Check sheet for the drawn part. Datum: minimum x, y, z corner. Units: mm. A direction names the side the tool comes from. Round coordinates to 2 decimals unless told otherwise and drop trailing zeros. Order: outer loops, then holes, each group sorted by start corner. A loop starts at its lowest first (then second) coordinate and runs counter-clockwise, first axis right, second up. Notation, with made-up numbers: (85.5, 88) -> (89.5, 88) arc R14 ccw to (89.5, 106) -> close; hole circle Ø6 at (64.25, 83.5). An arc over 180 degrees is marked (long way). Use CSV: the item, a comma, the result in double quotes.
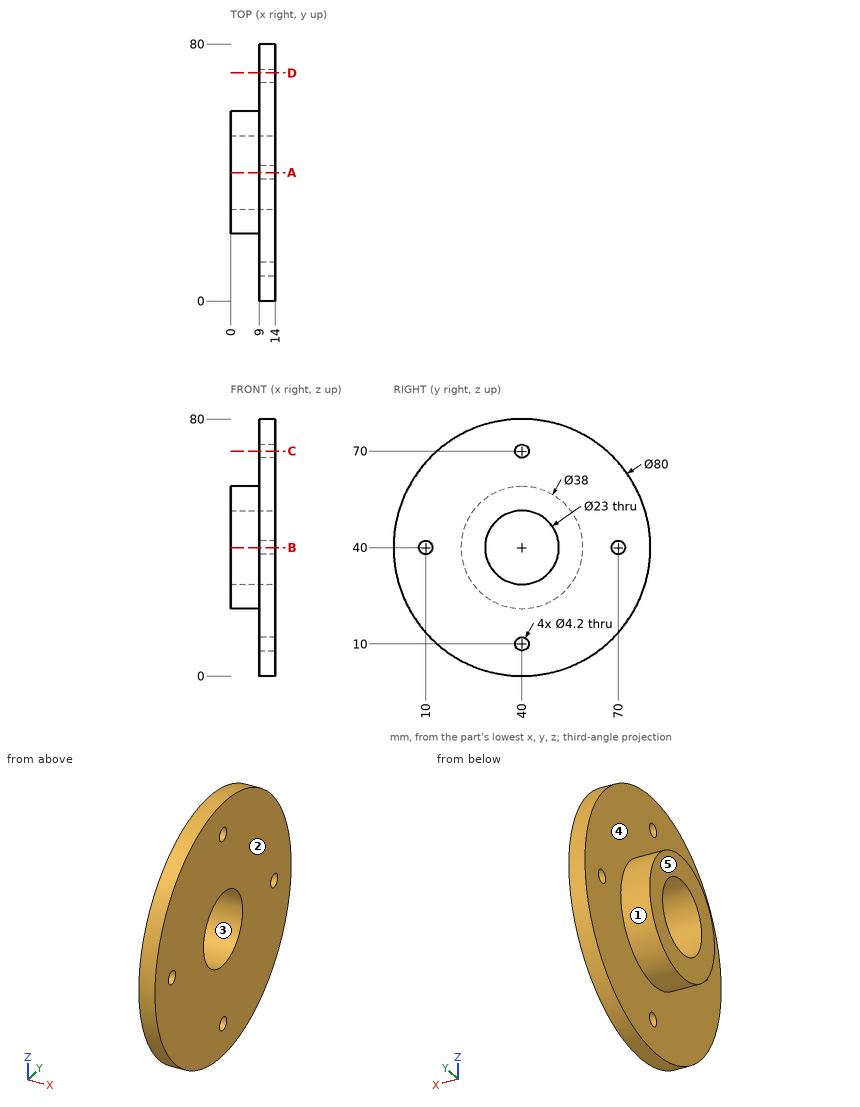
Q1. Access from +Z, -Z, +X, -X, +Y, -Y to the whole of each face (thin tool, end or side, straight path). Record for the marked faces 4 and 5.
Result sheet:
face 4,"-X"
face 5,"+Z, -Z, -X, +Y, -Y"
Q2. Sectioned sample at D-D, the plane y = 71. Enter the section's corners in (x, z).
Result sheet:
outline,"(9, 14.72) -> (14, 14.72) -> (14, 38.15) -> (9, 38.15) -> close; (9, 41.85) -> (14, 41.85) -> (14, 65.28) -> (9, 65.28) -> close"
Q3. Mould release check, pull along Z, two halves, no side actions. Record for the marked faces 1, 2 and 3: pulls with the +Z half, pulls with the -Z half, needs draft (parallel to the pull), parting line crosses it, or undercut.
Result sheet:
face 1,"parting line crosses it"
face 2,"needs draft"
face 3,"undercut"
Q4. Sectioned sample at A-A, the plane y = 40. Enter the section's corners in (x, z).
Result sheet:
outline,"(0, 21) -> (9, 21) -> (9, 12.1) -> (14, 12.1) -> (14, 28.5) -> (0, 28.5) -> close; (0, 51.5) -> (14, 51.5) -> (14, 67.9) -> (9, 67.9) -> (9, 59) -> (0, 59) -> close; (9, 0) -> (14, 0) -> (14, 7.9) -> (9, 7.9) -> close; (9, 72.1) -> (14, 72.1) -> (14, 80) -> (9, 80) -> close"
Q5. Go/stop test with flat-tipped pins: pin 1 (6 mm diameter, centred on y = 8.5, z = 35, fed in from -X); pin 2 (3.5 mm diameter, centred on y = 10, z = 40, fed in from -X); pin 3 (5 mm diameter, centred on x = 10, y = 22.5, fed in from +Z); pin 4 (3 mm diameter, centred on x = 6.5, z = 44, fed in from +Y). Record where each tip stops, or that it passes through.
Result sheet:
pin 1,"stops at x = 9"
pin 2,"passes through"
pin 3,"stops at z = 77.08"
pin 4,"stops at y = 58.83"
Q6. Scan lines: L1, parallel to Z at x = 12.05, y = 40; L2, parallel to Y at x = 3, z = 40; L3, parallel to X at y = 23, z = 66.5. Record each from-to range of solid material in increasing order.
Result sheet:
L1,"z = 0 to 7.9, 12.1 to 28.5, 51.5 to 67.9, 72.1 to 80"
L2,"y = 21 to 28.5, 51.5 to 59"
L3,"x = 9 to 14"
Q7. Sectioned sample at C-C, the plane z = 70. Enter the section's corners in (x, y), then the cut area to 3 significant figures.
Result sheet:
outline,"(9, 13.54) -> (14, 13.54) -> (14, 37.9) -> (9, 37.9) -> close; (9, 42.1) -> (14, 42.1) -> (14, 66.46) -> (9, 66.46) -> close"
area,"244 mm^2"
